Geometry check sheet. Reference: the model listing, model coordinates, mm. A direction names the side the tool comes from. Give positions to 0.01 mm unless a question says otherwise; leave off trailing zeros. Write each loop counter-clockwise with the first axis right and the second up, starting at its lowest first coordinate (ties: lowest second). Pieces come first, ordered by that corner, then holes.
(1) Cross-section at B-B (x = 1185.5). Record the boundary of the cut face in (y, z), and give its area (3 significant figures).
(2) Thickness scan on line 1 along Y through (x, z) = (537, 665); line 2 along X through (y, z) = (755, 552); line 3 along Z through (x, y) = (178, 329). Record the ranges inside material, lowest first.
(3) Depth check by flat-ended pin: P1, Ø1, axis at x = 1163.5, y = 99, coming from the +Z side; P2, Ø1, axis at x = 1679, z = 948, coming from the -Y side. Enter the tip coordinate at first touch or a pass-through.
(4) Cross-section at A-A (z = 784). Record the boundary of the cut face in (x, y).
(5) Cross-section at C-C (y = 159). Record the boundary of the cut face in (x, z), and give its area (3 significant figures).
(6) Tool access check on faces 1 (the cylindrical face through (2485.742, 784.964, 517.65)), 2 (the cylindrical face through (14.258, 252.8, 484.964)), 3 (the cylindrical face through (2484.964, 252.8, 485.742)), 4 (the flat face through (1233, 253, 500)). Record the directions out of +Z, -Z, +X, -X, +Y, -Y that give a thin tool (end or side, any length) a straight path to the whole face; none if there is none.
```python
from build123d import *

# Parameters (mm, degrees)
F0_W     = 2500
F0_H     = 800
F1_DEPTH = 500
F2_W     = 2500
F2_H     = 300
F3_DEPTH = 600
F4_R     = 50


with BuildPart() as f1:
    # F0 (on Top) → F1 (new body)
    with BuildSketch(Plane.XY):
        with Locations((1250, 400)):
            Rectangle(F0_W, F0_H)
    extrude(amount=F1_DEPTH)

    # F2 (on face) → F3 (join)
    with BuildSketch(Plane.XY.offset(500)):
        with Locations((1250, 650)):
            Rectangle(F2_W, F2_H)
    extrude(amount=F3_DEPTH)

    # F4
    f4_edges = [f1.edges().sort_by_distance(p)[0] for p in [
        (1250, 500, 500),
        (1250, 0, 500),
        (0, 0, 250),
        (0, 250, 500),
        (0, 800, 550),
        (1250, 500, 1100),
        (1250, 800, 1100),
        (2500, 500, 800),
        (2500, 250, 500),
        (2500, 0, 250),
        (2500, 800, 550),
        (2500, 650, 1100),
        (0, 650, 1100),
        (0, 500, 800),
    ]]
    fillet(f4_edges, radius=F4_R)


solid = f1.part
```
Reply:
1. outline: (0, 0) - (800, 0) - (800, 1050) arc R50 ccw to (750, 1100) - (550, 1100) arc R50 ccw to (500, 1050) - (500, 550) arc R50 cw to (450, 500) - (50, 500) arc R50 ccw to (0, 450) - close
1. area: 579,000 mm2
2. line 1: y = 500 to 800
2. line 2: x = 0.25 to 2499.75
2. line 3: z = 0 to 500
3. P1: stops at z = 500
3. P2: stops at y = 500
4. outline: (0, 550) arc R50 ccw to (50, 500) - (2450, 500) arc R50 ccw to (2500, 550) - (2500, 750) arc R50 ccw to (2450, 800) - (50, 800) arc R50 ccw to (0, 750) - close
5. outline: (0, 0) - (2500, 0) - (2500, 450) arc R50 ccw to (2450, 500) - (50, 500) arc R50 ccw to (0, 450) - close
5. area: 1,250,000 mm2
6. face 1: +Z, -Z, +X, +Y
6. face 2: +Z, -X, -Y
6. face 3: +Z, +X, -Y
6. face 4: +Z, +X, -X, -Y
